```python
from build123d import *

# Parameters (mm, degrees)
BOSS_EXTRUDE6_DEPTH = 12.7
SKETCH10_R          = 25.4
BOSS_EXTRUDE7_DEPTH = 25.4
SHELL14_T           = 2.5399999999999943
FILLET1_R           = 2.54
BOSS_EXTRUDE8_DEPTH = 25.4
SKETCH12_W          = 12.7
SKETCH12_H          = 2.5399999999999974
CUT_EXTRUDE6_DEPTH  = 25.4
CUT_EXTRUDE7_REACH  = 108.984
SKETCH15_W          = 25.4
SKETCH15_H          = 12.699999999999998


with BuildPart() as part:
    # Sketch9 → Boss-Extrude6 (new body)
    with BuildSketch(Plane(origin=(0, 0, 0), x_dir=(1, 0, 0), z_dir=(0, 1, 0))):
        with BuildLine():
            ThreePointArc((-63.5, 12.699999999999985), (-76.2, -1.232e-14), (-63.5, -12.700000000000014))
            ThreePointArc((-63.5, -12.700000000000014), (-35.34389302544592, -14.875381401189138), (-12.7, -31.75))
            ThreePointArc((-12.7, -31.75), (1.154e-14, -44.45000000000002), (12.7, -31.75))
            ThreePointArc((12.7, -31.75), (35.34389302544593, -14.875381401189138), (63.5, -12.700000000000001))
            ThreePointArc((63.5, -12.700000000000001), (76.2, 1.68e-15), (63.5, 12.700000000000001))
            ThreePointArc((63.5, 12.700000000000001), (35.34389302544591, 14.87538140118913), (12.7, 31.75))
            ThreePointArc((12.7, 31.75), (4.06e-15, 44.44999999999999), (-12.7, 31.75))
            ThreePointArc((-12.7, 31.75), (-35.34389302544592, 14.87538140118913), (-63.5, 12.699999999999985))
        make_face()
    extrude(amount=BOSS_EXTRUDE6_DEPTH)

    # Sketch10 → Boss-Extrude7 (add)
    with BuildSketch(Plane(origin=(0, 12.7, 0), x_dir=(1, 0, 0), z_dir=(0, 1, 0))):
        with Locations(Location((0, 0, 0), (0, 0, 270))):
            Circle(SKETCH10_R)
    extrude(amount=BOSS_EXTRUDE7_DEPTH)

    # Shell14
    shell14_openings = [part.faces().sort_by_distance(p)[0] for p in [
        (0, 38.1, 0),
    ]]
    offset(amount=SHELL14_T, openings=shell14_openings, kind=Kind.INTERSECTION)

    # Fillet1
    # the kernel refuses this fillet: 2.54 mm, written as the material it adds along each edge
    with BuildSketch(Plane(origin=(15.213395442859193, 15.239999999999993, 32.65011060386543), x_dir=(-0.08244746024425967, 0, 0.9965954125417552), z_dir=(0, -1, 0))) as fillet1_piece_1:
        with BuildLine():
            CenterArc((0.7740627209529523, -2.5393019901274583), FILLET1_R, 91.3432643866729, 32.987937528232266)
            ThreePointArc((-0.6584359095530802, -0.44179211563381704), (-0.33012530713560906, -0.2195437625751302), (0, 0))
            ThreePointArc((0, 0), (0.357259717362898, -0.00418805923524796), (0.7145194347258012, 0))
        make_face()
    extrude(amount=17.779999999999987)
    with BuildSketch(Plane(origin=(-15.213395442859223, 15.239999999999993, 32.65011060386536), x_dir=(-0.623740024012636, 0, -0.7816318714361103), z_dir=(0, -1, 0))) as fillet1_piece_2:
        with BuildLine():
            CenterArc((0.7720512245924565, -2.5399142898215286), FILLET1_R, 89.52930650878288, 32.98793752823278)
            ThreePointArc((-0.5933344507841877, -0.3981108540515074), (-0.2943337523500303, -0.20253317683271896), (0, 0))
            ThreePointArc((0, 0), (0.396458736952872, 0.00162849339096533), (0.7929174739057625, 3e-17))
        make_face()
    extrude(amount=17.779999999999987)
    with BuildSketch(Plane(origin=(-15.213395442859191, 15.239999999999993, -32.6501106038654), x_dir=(-0.6237400240126415, 0, 0.781631871436106), z_dir=(0, -1, 0))) as fillet1_piece_3:
        with BuildLine():
            CenterArc((0.7720512245925322, 2.5399142898215272), FILLET1_R, 237.48275596298424, 32.987937528232294)
            ThreePointArc((-0.593334450784115, 0.3981108540515081), (-0.2943337523499901, 0.20253317683272415), (0, 0))
            ThreePointArc((0, 0), (0.3964587369529053, -0.00162849339097196), (0.7929174739058125, 2e-17))
        make_face()
    extrude(amount=17.779999999999987)
    with BuildSketch(Plane(origin=(15.21339544285919, 15.239999999999993, -32.65011060386541), x_dir=(-0.08244746024426708, 0, -0.9965954125417545), z_dir=(0, -1, 0))) as fillet1_piece_4:
        with BuildLine():
            CenterArc((0.7740627209529621, 2.539301990127459), FILLET1_R, 235.66879808509486, 32.987937528232465)
            ThreePointArc((-0.6584359095530695, 0.44179211563381504), (-0.330125307135611, 0.21954376257513125), (0, 0))
            ThreePointArc((0, 0), (0.3572597173629123, 0.00418805923525002), (0.714519434725823, 0))
        make_face()
    extrude(amount=17.779999999999987)
    # the kernel refuses this fillet: 2.54 mm, written as the material it takes off along each edge
    with BuildSketch(Plane(origin=(63.22420496202578, 15.929515824336315, 15.23750429358524), x_dir=(-0.9786320251398054, 0, -0.2056194528024121), z_dir=(0, -1, 0))) as fillet1_2_piece_1:
        with BuildLine():
            CenterArc((0.25185838779454184, 2.5399917904261593), FILLET1_R, 258.13423637706234, 11.720089907990712)
            ThreePointArc((-0.2704150223235917, 0.05426644657105567), (-0.13533027474319617, 0.02652148032641584), (0, 0))
            ThreePointArc((0, 0), (0.12270024020757794, 0.00015598190298779), (0.2454004804151519, 0))
        make_face()
    extrude(amount=19.15903164867263, mode=Mode.SUBTRACT)
    with BuildSketch(Plane(origin=(-63.22420496202586, 15.929515824336706, 15.237504293585257), x_dir=(-0.9999590590960623, 0, 0.009048764098899606), z_dir=(0, -1, 0))) as fillet1_2_piece_2:
        with BuildLine():
            CenterArc((0.2528224689234374, 2.5398960101039973), FILLET1_R, 258.79837316015426, 11.720089907990541)
            ThreePointArc((-0.24060352948943128, 0.04828392470822683), (-0.12027107442804234, 0.02429489521037388), (0, 0))
            ThreePointArc((0, 0), (0.1379031648673247, -0.00062393937600912), (0.27580632973464947, 0))
        make_face()
    extrude(amount=19.159031648673412, mode=Mode.SUBTRACT)
    with BuildSketch(Plane(origin=(-63.22420496202585, 15.92951582433667, -15.237504293585229), x_dir=(-0.9999590590960623, 0, -0.00904876409889914), z_dir=(0, -1, 0))) as fillet1_2_piece_3:
        with BuildLine():
            CenterArc((0.2528224689234528, -2.5398960101039973), FILLET1_R, 89.48153693185522, 11.720089907991053)
            ThreePointArc((-0.2406035294894384, -0.04828392470823043), (-0.12027107442802101, -0.02429489521037413), (0, 0))
            ThreePointArc((0, 0), (0.1379031648673247, 0.00062393937600918), (0.2758063297346637, 0))
        make_face()
    extrude(amount=19.15903164867334, mode=Mode.SUBTRACT)
    with BuildSketch(Plane(origin=(63.22420496202587, 15.929515824336635, -15.237504293585246), x_dir=(0.9999590590960625, 0, -0.00904876409889984), z_dir=(0, -1, 0))) as fillet1_2_piece_4:
        with BuildLine():
            CenterArc((0.25282246892342264, 2.539896010103998), FILLET1_R, 258.79837316015426, 11.720089907990712)
            ThreePointArc((-0.24060352948944552, 0.04828392470822666), (-0.12027107442801392, 0.02429489521037056), (0, 0))
            ThreePointArc((0, 0), (0.13790316486732473, -0.00062393937600909), (0.2758063297346424, 0))
        make_face()
    extrude(amount=19.15903164867327, mode=Mode.SUBTRACT)

    # Sketch11 → Boss-Extrude8 (add)
    with BuildSketch(Plane(origin=(0, 0, 0), x_dir=(1, 0, 0), z_dir=(0, 1, 0))):
        Polygon((8.889999999999997, 14.605), (8.890000000000002, -14.605), (-8.889999999999999, -14.604999999999997), (-8.890000000000002, 14.605), align=None)
        Polygon((-6.350000000000001, 12.065), (6.349999999999998, 12.065), (6.3500000000000005, -12.065), (-6.349999999999999, -12.065), align=None, mode=Mode.SUBTRACT)
    extrude(amount=BOSS_EXTRUDE8_DEPTH)

    # Sketch12 → Cut-Extrude6 (cut)
    with BuildSketch(Plane(origin=(0, 25.4, 0), x_dir=(1, 0, 0), z_dir=(0, 1, 0))):
        with Locations((8.9e-16, -13.334999999999997)):
            Rectangle(SKETCH12_W, SKETCH12_H)
    extrude(amount=-CUT_EXTRUDE6_DEPTH, mode=Mode.SUBTRACT)

    # Sketch15 → Cut-Extrude7 (cut, up to next)
    with BuildSketch(Plane.XY.offset(14.604999999999999), mode=Mode.PRIVATE) as cut_extrude7_sk1:
        with Locations((1.865e-14, 6.349999999999999)):
            Rectangle(SKETCH15_W, SKETCH15_H)
    cut_extrude7_tool1 = extrude(cut_extrude7_sk1.sketch, amount=CUT_EXTRUDE7_REACH, mode=Mode.PRIVATE) & part.part
    add(cut_extrude7_tool1.solids().sort_by_distance((0, 6.35, 14.605))[0], mode=Mode.SUBTRACT)


solid = part.part
```
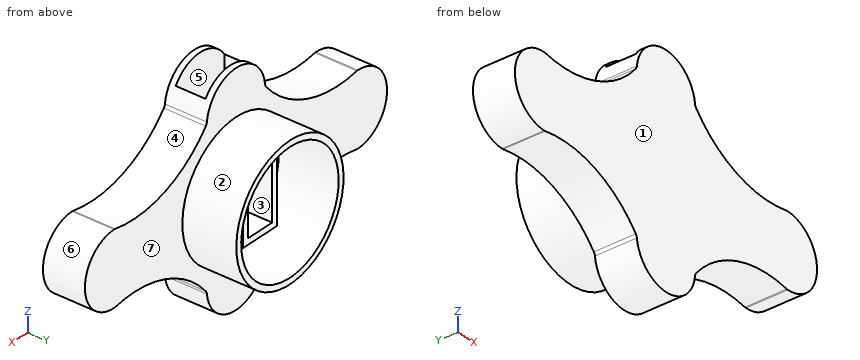
The model under review builds one solid part; all positions refer to its coordinate system, in mm. Face numbers are marked on the shaded views. A direction names the side the tool comes from. Round coordinates to 2 decimals unless told otherwise and drop trailing zeros. Loops run counter-clockwise (first coordinate to the right, second up) from the corner with the lowest first, then second, coordinate; pieces in that order, holes last. Notation, with made-up numbers: M 65,41 L 99,41 A35 ccw 99,74 Z; hole C 55,68 d8. An arc over 180 degrees is marked long. Put each result on its own line as item: value.
Q1. To check wall thickness, follow L1, parallel to X at y = 21.25, z = 0; L2, parallel to X at y = 27, z = 0; L3, parallel to Z at x = -1.5, y = 24.5 (3 decimals). State the ranges of each line that lie inside material, in increasing order.
Result set:
L1: x = -27.94 to -25.4, -8.89 to -6.35, 6.35 to 8.89, 25.4 to 27.94
L2: x = -27.94 to -25.4, 25.4 to 27.94
L3: z = -27.9 to -25.356, -14.605 to -12.065, 25.356 to 27.9
Q2. Consider section C-C, the plane x = 0. Give the boundary of the cut face in (y, z) (3 decimals), then the cut area to 3 significant figures.
Result set:
outline: M -2.54,-46.99 L 15.24,-46.99 L 15.24,-27.94 L 38.1,-27.94 L 38.1,-25.4 L 12.7,-25.4 L 12.7,-44.45 L 0,-44.45 L 0,-14.605 L 25.4,-14.605 L 25.4,-12.065 L 0,-12.065 L 0,46.99 L -2.54,46.99 Z; M 12.7,25.4 L 38.1,25.4 L 38.1,27.94 L 15.24,27.94 L 15.24,46.99 L 12.7,46.99 Z
area: 561 mm²
Q3. Consider section A-A, the plane y = 20. Give the boundary of the cut face in (x, z) (3 decimals).
Result set:
outline: C 0,0 d55.88; M -8.89,-14.605 L 8.89,-14.605 L 8.89,14.605 L 6.35,14.605 L 6.35,-12.065 L -6.35,-12.065 L -6.35,14.605 L -8.89,14.605 Z; hole C 0,0 d50.8
Q4. Machinability: for the marked faces 5, 6 and 7, which of the approach directions +Z, -Z, +X, -X, +Y, -Y give a long, thin tool a straight path to every point of the face, cutting with its end or side? Answer none if there is none.
Result set:
face 5: none
face 6: +X, +Y, -Y
face 7: +Y
Q5. For pin 1 (5 mm diameter, centred on y = 14, z = -33, fed in from +X); pin 2 (2 mm diameter, centred on x = 7.5, y = 11.5, fed in from +Z) (3 decimals); pin 3 (9 mm diameter, centred on x = -0.5, z = -1.5, fed in from +Y), all flat-tipped, find the tip position at first contact; note any pin that passes through.
Result set:
pin 1: stops at x = 17
pin 2: stops at z = 14.605
pin 3: stops at y = 0
Q6. Mouldability with a two-part tool opening along X and no side actions: class the marked faces 1, 2, 3 and 4 as released by +X, released by -X, zero draft, split by the parting line, or undercut.
Result set:
face 1: zero draft
face 2: split by the parting line
face 3: undercut
face 4: undercut
Q7. Consider section D-D, the plane x = 69.5. Give the boundary of the cut face in (y, z), then the cut area to 3 significant figures.
Result set:
outline: M -2.54,-14.01 L 15.24,-14.01 L 15.24,14.01 L -2.54,14.01 Z; hole M 0,-11.19 L 12.7,-11.19 L 12.7,11.19 L 0,11.19 Z
area: 214 mm²
